CAD build for the part. Positions are in the model's coordinates, mm. A direction names the side the tool comes from. Coordinates: 2 decimals unless noted, no trailing zeros. Write each loop counter-clockwise with the first axis right and the second up, starting at its lowest first coordinate (ties: lowest second). Pieces come first, ordered by that corner, then holes. Notation, with made-up numbers: (65.5, 46.5) -> (101.5, 46.5) arc R27 cw to (101.5, 65.5) -> close; hole circle Ø3 at (-16, -6.5). An arc over 180 degrees is marked (long way). Answer as CSV lines item,"result". Start each with the question number.
```python
from build123d import *

# Parameters (mm, degrees)
EXTRUSION1_DEPTH = 20
ESQUISSE2_W      = 54
ESQUISSE2_H      = 35
EXTRUSION2_DEPTH = 27
ESQUISSE4_W      = 10
ESQUISSE4_H      = 5
EXTRUSION4_DEPTH = 77.66


with BuildPart() as part:
    # Esquisse1 → Extrusion1 (new body)
    with BuildSketch(Plane.XY):
        Polygon((0, 0), (-8, 0), (-8, 20.66), (-42, 20.66), (-42, 0), (-50, 0), (-50, -3), (-52, -3), (-52, 73.66), (2, 73.66), (2, -3), (0, -3), align=None)
    extrude(amount=EXTRUSION1_DEPTH)

    # Esquisse2 → Extrusion2 (add)
    with BuildSketch(Plane.XY.offset(20)):
        with Locations((-25, 56.16)):
            Rectangle(ESQUISSE2_W, ESQUISSE2_H)
    extrude(amount=EXTRUSION2_DEPTH)

    # Esquisse4 → Extrusion4 (cut, through all)
    with BuildSketch(Plane(origin=(0, 73.66, 0), x_dir=(1, 0, 0), z_dir=(0, 1, 0))):
        with Locations((-25, -44.5)):
            Rectangle(ESQUISSE4_W, ESQUISSE4_H)
    extrude(amount=-EXTRUSION4_DEPTH, mode=Mode.SUBTRACT)


solid = part.part
```
1. Cut at D-D (x = -46). Give the cut face in (y, z).
2. Flat gauge pins, fed straight in: P1, Ø22, axis at x = -20, z = 13.5, coming from the -Y side; P2, Ø3, axis at x = -23.5, y = 57.5, coming from the +Z side; P3, Ø2, axis at x = -42.5, z = 29.5, coming from the -Y side. Where does each tip first touch, or does it go through?
3. Wall check: line 1 (X direction, y = 5, z = 5.5); line 2 (Y direction, x = -28, z = 25); line 3 (Y direction, x = -29.5, z = 6). Give the ranges that are in metal, low to high.
4. Tool access for faces 1 (the face through (-25, 20.66, 10)), 2 (the face through (-30, 56, 45)), 3 (the face through (-25, 38.66, 33)): list every direction of +Z, -Z, +X, -X, +Y, -Y with a clear straight run to the whole face (end or side of a thin tool).
5. Cut at A-A (z = 43.5). Give the cut face in (x, y), then the cut area to 3 significant figures.
6. Cut at B-B (y = 59.5). Give the cut face in (x, z), then the cut area to 3 significant figures.
7. Mould opens along X. For faces 4 (the face through (1, -3, 10)), 5 (the face through (-25, 56, 42)), 6 (the face through (2, 43, 18)) say: pulls with the +X half, pulls with the -X half, needs draft (parallel to the pull), parting line crosses it, or undercut.
8. Cut at C-C (z = 17). Give the cut face in (x, y).
Geometry check:
1,outline,"(0, 0) -> (73.66, 0) -> (73.66, 47) -> (38.66, 47) -> (38.66, 20) -> (0, 20) -> close"
2,P1,"y = 20.66"
2,P2,"z = 42"
2,P3,"y = 38.66"
3,line 1,"-52 to -42, -8 to 2"
3,line 2,"38.66 to 73.66"
3,line 3,"20.66 to 73.66"
4,face 1,"+Z, -Z, -Y"
4,face 2,"+Z, +Y, -Y"
4,face 3,"+Z, +X, -X, -Y"
5,outline,"(-52, 38.66) -> (-30, 38.66) -> (-30, 73.66) -> (-52, 73.66) -> close; (-20, 38.66) -> (2, 38.66) -> (2, 73.66) -> (-20, 73.66) -> close"
5,area,"1,540 mm²"
6,outline,"(-52, 0) -> (2, 0) -> (2, 47) -> (-20, 47) -> (-20, 42) -> (-30, 42) -> (-30, 47) -> (-52, 47) -> close"
6,area,"2,490 mm²"
7,face 4,"needs draft"
7,face 5,"undercut"
7,face 6,"pulls with the +X half"
8,outline,"(-52, -3) -> (-50, -3) -> (-50, 0) -> (-42, 0) -> (-42, 20.66) -> (-8, 20.66) -> (-8, 0) -> (0, 0) -> (0, -3) -> (2, -3) -> (2, 73.66) -> (-52, 73.66) -> close"
